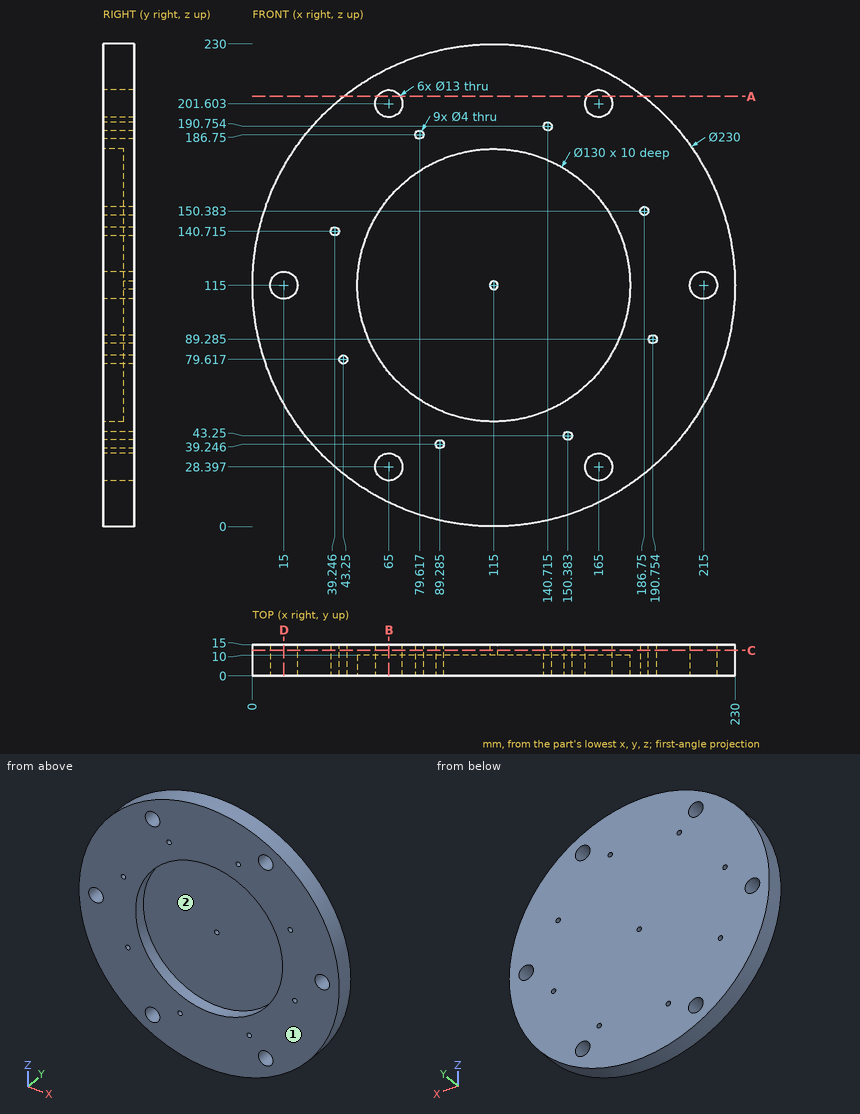
Print and shaded views of the part. All mm, measured from the part's lowest x, y and z. Round coordinates to 2 decimals unless told otherwise and drop trailing zeros. Write each loop counter-clockwise with the first axis right and the second up, starting at its lowest first coordinate (ties: lowest second). Pieces come first, ordered by that corner, then holes. Notation, with made-up numbers: (36.5, 71.25) - (74.5, 71.25) arc R24 ccw to (74.5, 84.25) - close; hole circle Ø11 at (-7.5, 51). An arc over 180 degrees is marked (long way). Use CSV: the item, a comma, the result in double quotes. Start each with the question number.
Item 1: Pin check, flat tips, straight feed: P1, Ø3.5, axis at x = 43.25, z = 79.62, coming from the -Y side; P2, Ø1.5, axis at y = 4.5, z = 80.5, coming from the -X side; P3, Ø6, axis at x = 205, y = 9.5, coming from the +Z side (1 decimal); P4, Ø8, axis at y = 2.5, z = 158, coming from the -X side (1 decimal). Stop position of each tip, or through.
Item 2: Band-saw the part on D-D (x = 15). Write the cut outline in (y, z).
Item 3: Drill centre lines: L1, parallel to X at y = 9.75, z = 115; L2, parallel to Z at x = 65, y = 10.75; L3, parallel to X at y = 4.5, z = 149 (1 decimal). Where is each one in solid material? Low to high. Write a range as [from, to].
Item 4: Band-saw the part on B-B (x = 65). Write the cut outline in (y, z), and give its area (3 significant figures).
Item 5: Two-plate mould, pull along X, no slides. Class the marked faces 1 and 2: released by +X, released by -X, zero draft, split by the parting line, or undercut.
Item 6: Band-saw the part on A-A (z = 205). Write the cut outline in (x, y), and give its area (4 significant figures).
Item 7: Band-saw the part on C-C (y = 12.25). State how many separate pieces and enclosed holes the cut face has, and give its area (3 significant figures).
Checked values:
1,P1,"passes through"
1,P2,"stops at x = 5.06"
1,P3,"stops at z = 190.2"
1,P4,"stops at x = 6.8"
2,outline,"(0, 58.21) - (15, 58.21) - (15, 108.5) - (0, 108.5) - close; (0, 121.5) - (15, 121.5) - (15, 171.79) - (0, 171.79) - close"
3,L1,"x = [0, 8.5], [21.5, 50], [180, 208.5], [221.5, 230]"
3,L2,"z = [11.44, 21.9], [34.9, 195.1], [208.1, 218.56]"
3,L3,"x = [5.1, 59.6], [170.4, 185.3], [188.2, 224.9]"
4,outline,"(0, 11.44) - (15, 11.44) - (15, 21.9) - (0, 21.9) - close; (0, 34.9) - (15, 34.9) - (15, 195.1) - (0, 195.1) - (0, 156.53) - (10, 156.53) - (10, 73.47) - (0, 73.47) - close; (0, 208.1) - (15, 208.1) - (15, 218.56) - (0, 218.56) - close"
4,area,"1,890 mm²"
5,face 1,"zero draft"
5,face 2,"undercut"
6,outline,"(43.41, 0) - (59.46, 0) - (59.46, 15) - (43.41, 15) - close; (70.54, 0) - (159.46, 0) - (159.46, 15) - (70.54, 15) - close; (170.54, 0) - (186.59, 0) - (186.59, 15) - (170.54, 15) - close"
6,area,"1,815 mm²"
7,separate pieces,"1"
7,enclosed holes,"15"
7,area,"40,600 mm²"
